Can you work these out from the drawing? Everything is in mm from the part's minimum corner. A direction names the side the tool comes from. Round coordinates to 2 decimals unless told otherwise and drop trailing zeros. Order: outer loops, then holes, each group sorted by start corner. A loop starts at its lowest first (then second) coordinate and runs counter-clockwise, first axis right, second up. Notation, with made-up numbers: M -9.75,10.25 L 14.25,10.25 A23 cw 14.25,43.25 Z; hole C -13.5,18 d4. An arc over 180 degrees is marked long. Write item = value, one per line. Start each with the question number.
Item 1: I'm going to push flat-ended pins straight in: P1, Ø0.7, axis at y = 2.5, z = 0.5, coming from the +X side; P2, Ø1, axis at x = 1, y = 2, coming from the +Z side; P3, Ø0.7, axis at y = 2.5, z = 1, coming from the -X side. Where does each tip first touch, or does it pass through?
Item 2: I want a section at C-C, the plane y = 1.8. List the corners of the cut face in (x, z) for me.
Item 3: I want a section at A-A, the plane z = 1.25. List the corners of the cut face in (x, y) for me.
Item 4: Please list where these lines run through material, in increasing order: L1, parallel to Y at x = 0.35, z = 6.25; L2, parallel to Y at x = 0.25, z = 2.5 (1 decimal); L3, parallel to Z at x = 1.65, y = 0.2 (1 decimal).
Item 5: I want a section at D-D, the plane x = 2.3. List the corners of the cut face in (y, z) for me (1 decimal).
Item 6: I want a section at B-B, the plane x = 1.3. List the corners of the cut face in (y, z) for me (1 decimal).
Item 7: For the marked faces 1 and 2, which set-ups out of +Z, -Z, +X, -X, +Y, -Y let a thin tool reach every point of the face, with its end or its side?
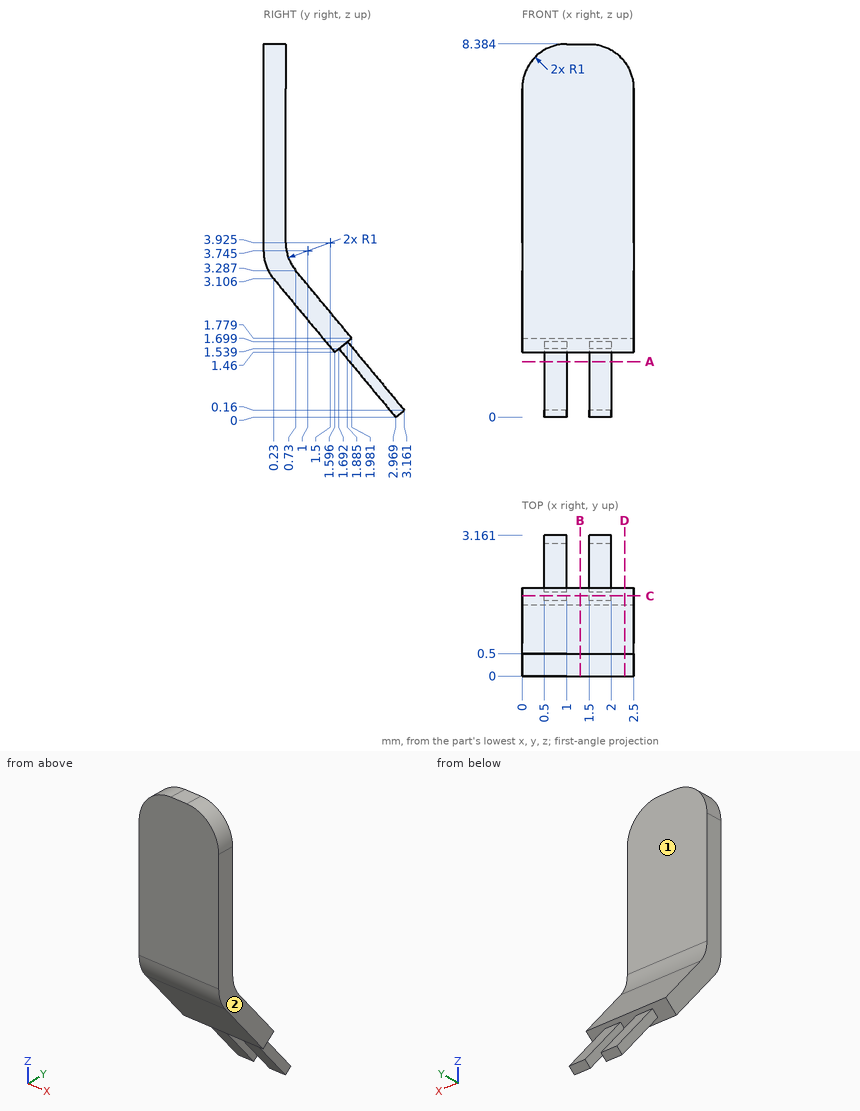
Filled in:
q1.P1 = 2
q1.P2 = 2.36
q1.P3 = 0.5
q2.outline = M 0,1.63 L 0.5,1.63 L 0.5,1.41 L 1,1.41 L 1,1.63 L 1.5,1.63 L 1.5,1.41 L 2,1.41 L 2,1.63 L 2.5,1.63 L 2.5,2 L 0,2 Z
q3.outline = M 0.5,1.93 L 1,1.93 L 1,2.26 L 0.5,2.26 Z; M 1.5,1.93 L 2,1.93 L 2,2.26 L 1.5,2.26 Z
q4.L1 = 0 to 0.5
q4.L2 = 0.7 to 1.4
q4.L3 = 3.1 to 8.4
q5.outline = M 0,3.7 A1 ccw 0.2,3.1 L 1.6,1.5 L 2,1.8 L 0.7,3.3 A1 cw 0.5,3.9 L 0.5,8 L 0,8 Z
q6.outline = M 0,3.7 A1 ccw 0.2,3.1 L 1.6,1.5 L 2,1.8 L 0.7,3.3 A1 cw 0.5,3.9 L 0.5,8.4 L 0,8.4 Z
q7.face_1 = +Z, +X, -X, +Y
q7.face_2 = +Z, -Z, +X, +Y, -Y
